Build history of the part. All positions in model axes, mm. Face numbers are marked on the shaded views. A direction names the side the tool comes from. Round coordinates to 2 decimals unless told otherwise and drop trailing zeros. Write each loop counter-clockwise with the first axis right and the second up, starting at its lowest first coordinate (ties: lowest second). Pieces come first, ordered by that corner, then holes. Notation, with made-up numbers: (28.5, -6.5) - (32.5, -6.5) arc R11 ccw to (32.5, 11.5) - close; hole circle Ø5 at (35, -7.5). An arc over 180 degrees is marked (long way). One line per question, with ' | ' between items.
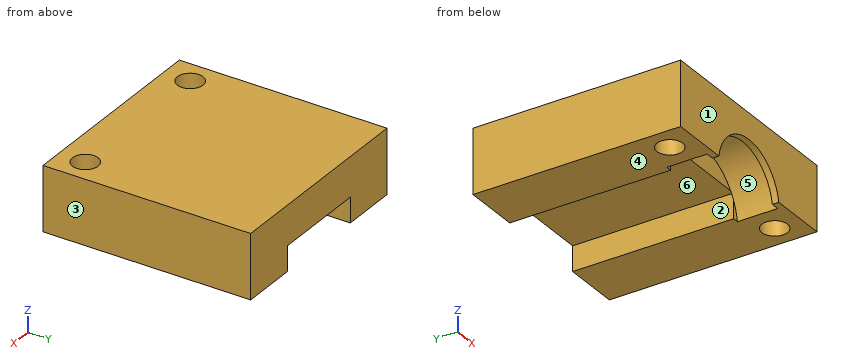
from build123d import *

# Parameters (mm, degrees)
F1_DEPTH = 2.5
F2_R     = 1.6
F3_DEPTH = 12.5
F6_DEPTH = 20
F9_DEPTH = 0.8


with BuildPart() as f1:
    # F0 (on Front) → F1 (new body, symmetric)
    with BuildSketch(Plane.XZ):
        with BuildLine():
            Line((13, 4), (-13, 4))
            Line((-13, 4), (-13, -4))
            Line((-13, -4), (-6.7260686883, -4))
            ThreePointArc((-6.7260686883, -4), (0, 1.8), (6.7260686883, -4))
            Line((6.7260686883, -4), (13, -4))
            Line((13, -4), (13, 4))
        make_face()
    extrude(amount=F1_DEPTH, both=True)

    # F2 (on Top) → F3 (cut, symmetric)
    with BuildSketch(Plane.XY):
        with Locations((10, 0)):
            Circle(F2_R)
        with Locations((-10, 0)):
            Circle(F2_R)
    extrude(amount=F3_DEPTH, both=True, mode=Mode.SUBTRACT)

    # F5 (on offset) → F6 (join)
    with BuildSketch(Plane(origin=(0, 2.5, 0), x_dir=(-1, 0, 0), z_dir=(0, 1, 0))):
        Polygon((13, 4), (-13, 4), (-13, -4), (-6, -4), (-6, -0.9), (6, -0.9), (6, -4), (13, -4), align=None)
    extrude(amount=F6_DEPTH)

    # F8 (on offset) → F9 (join)
    with BuildSketch(Plane.XZ.offset(2.5)):
        with BuildLine():
            Line((13, 4), (-13, 4))
            Line((-13, 4), (-13, -4))
            Line((-13, -4), (-5.7131427428, -4))
            ThreePointArc((-5.7131427428, -4), (0, 0.8), (5.7131427428, -4))
            Line((5.7131427428, -4), (13, -4))
            Line((13, -4), (13, 4))
        make_face()
    extrude(amount=F9_DEPTH)


solid = f1.part
Q1. Saw through at D-D, the plane x = -2. List the corners of the cut face in (y, z).
Found:
outline: (-3.3, 0.44) - (-2.5, 0.44) - (-2.5, 1.5) - (2.5, 1.5) - (2.5, -0.9) - (22.5, -0.9) - (22.5, 4) - (-3.3, 4) - close
Q2. Saw through at B-B, the plane x = 10. List the corners of the cut face in (y, z), then the cut area to 3 significant figures.
Found:
outline: (-3.3, -4) - (-1.6, -4) - (-1.6, 4) - (-3.3, 4) - close; (1.6, -4) - (22.5, -4) - (22.5, 4) - (1.6, 4) - close | area: 181 mm^2
Q3. Saw through at A-A, the plane y = 0. List the corners of the cut face in (x, z), then the cut area to 3 significant figures.
Found:
outline: (-13, -4) - (-11.6, -4) - (-11.6, 4) - (-13, 4) - close; (-8.4, -4) - (-6.73, -4) arc R6.8 cw to (6.73, -4) - (8.4, -4) - (8.4, 4) - (-8.4, 4) - close; (11.6, -4) - (13, -4) - (13, 4) - (11.6, 4) - close | area: 97.7 mm^2
Q4. Pull direction X, two halves, no side cores. Call the marked faces 1, 2 and 3: +X half, -X half, draft (parallel to the pull), parting line (faces both ways), or undercut.
Found:
face 1: draft | face 2: undercut | face 3: +X half
Q5. Drill centre lines: L1, parallel to Y at x = 10, z = -1.5; L2, parallel to X at y = 16.5, z = -1; L3, parallel to X at y = 0.25, z = 3.5. Where is each one in solid material? Low to high. Write a range as from..to.
Found:
L1: -3.3..-1.6, 1.6..22.5 | L2: -13..-6, 6..13 | L3: -13..-11.58, -8.42..8.42, 11.58..13
Q6. Which spindle directions (+Z, -Z, +X, -X, +Y, -Y) get a long thin tool onto all of the face, cutting with end or side? Do the marked faces 4, 5 and 6. Say none if no direction does.
Found:
face 4: -Z, +X, -X, +Y, -Y | face 5: -Z | face 6: -Z, +Y
Q7. Drop flat-ended pins along their axis: pin 1 (1.9 mm diameter, centred on x = 10, y = 0, fed in from +Z); pin 2 (9.5 mm diameter, centred on x = -1, y = 14.5, fed in from -Z). Give the stop position or say it passes through.
Found:
pin 1: through | pin 2: z = -0.9
Q8. Saw through at C-C, the plane y = 9. List the corners of the cut face in (x, z).
Found:
outline: (-13, -4) - (-6, -4) - (-6, -0.9) - (6, -0.9) - (6, -4) - (13, -4) - (13, 4) - (-13, 4) - close
